Build history of the part. All positions in model axes, mm. A direction names the side the tool comes from. Round coordinates to 2 decimals unless told otherwise and drop trailing zeros. Write each loop counter-clockwise with the first axis right and the second up, starting at its lowest first coordinate (ties: lowest second). Pieces come first, ordered by that corner, then holes.
1) Which spindle directions (+Z, -Z, +X, -X, +Y, -Y) get a long thin tool onto all of the face, cutting with end or side? Do faces 1 (the flat face through (0.021, 7.127, -39.964)), 2 (the flat face through (0, 5, 2)), 3 (the flat face through (0.02, 0.58, -14.67)). Say none if no direction does.
2) Pull direction Z, two halves, no side cores. Call faces 4 (the flat face through (-1.5, 4, -14)), 5 (the cylindrical face through (-0.02, 0.07, 12.5)), 6 (the cylindrical face through (0, 0, 16)): +Z half, -Z half, draft (parallel to the pull), parting line (faces both ways), or undercut.
3) Wall check: probe 1 along Y at (x, z) = (0.1, 11); probe 2 along Z at (x, y) = (0.6, 0.5); probe 3 along Y at (x, z) = (0.35, 3). Give the ranges that are in metal, low to high.
4) Saw through at D-D (y = 3.5). Write the cut outline in (x, z), plus the area to 3 significant figures.
5) Saw through at A-A (x = -0.35). Write the cut outline in (y, z).
6) Saw through at B-B (y = 0). Write the cut outline in (x, z).
7) Flat gauge pins, fed straight in: pin 1 (3 mm diameter, centred on y = 3.5, z = -33.5, fed in from -X); pin 2 (1.5 mm diameter, centred on x = 0, y = 11, fed in from -Z); pin 3 (1.5 mm diameter, centred on x = 0.5, z = -2, fed in from +Y). Where does each tip first touch, or does it go through?
8) Saw through at C-C (z = 7.5). Write the cut outline in (x, y), plus the area to 3 significant figures.
from build123d import *

# Parameters (mm, degrees)
SKETCH1_R           = 5
SKETCH1_R_2         = 1.5
BOSS_EXTRUDE1_DEPTH = 1.5
BOSS_EXTRUDE2_DEPTH = 3
CUT_EXTRUDE1_DEPTH  = 3
CUT_EXTRUDE2_DEPTH  = 3


with BuildPart() as part:
    # Sketch1 → Boss-Extrude1 (new body, symmetric)
    with BuildSketch(Plane(origin=(0, 0, 0), x_dir=(0, 0, -1), z_dir=(1, 0, 0))):
        with BuildLine():
            ThreePointArc((-6, 0), (-7.464466094, -3.535533906), (-11, -5))
            Line((-11, -5), (11, -5))
            ThreePointArc((11, -5), (6, 0), (11, 5))
            Line((11, 5), (-11, 5))
            ThreePointArc((-11, 5), (-7.464466094, 3.535533906), (-6, 0))
        make_face()
        with Locations((-11, 0)):
            Circle(SKETCH1_R)
        with Locations((-11, 0)):
            Circle(SKETCH1_R_2, mode=Mode.SUBTRACT)
        with Locations((11, 0)):
            Circle(SKETCH1_R)
        with Locations((11, 0)):
            Circle(SKETCH1_R_2, mode=Mode.SUBTRACT)
    extrude(amount=BOSS_EXTRUDE1_DEPTH, both=True)

    # Sketch2 → Boss-Extrude2 (add)
    with BuildSketch(Plane(origin=(1.5, 0, 0), x_dir=(0, 0, -1), z_dir=(1, 0, 0))):
        with BuildLine():
            Line((34.743210425, 5.347223248), (34.979783381, 4.763328363))
            Line((34.979783381, 4.763328363), (44.247956153, 8.518454657))
            Line((44.247956153, 8.518454657), (40.196320101, 18.518454657))
            Line((40.196320101, 18.518454657), (6.830898124, 5))
            Line((6.830898124, 5), (11, 5))
            ThreePointArc((11, 5), (13.272352736, 4.453808824), (15.048249866, 2.934565218))
            Line((15.048249866, 2.934565218), (28.023691746, 8.191742029))
            Line((28.023691746, 8.191742029), (34.743210425, 5.347223248))
        make_face()
    extrude(amount=-BOSS_EXTRUDE2_DEPTH)

    # Sketch3 → Cut-Extrude1 (cut)
    with BuildSketch(Plane(origin=(1.5, 0, 0), x_dir=(0, 0, -1), z_dir=(1, 0, 0))):
        Polygon((40.196320101, 18.518454657), (35.196320101, 16.492636631), (42.222138127, 13.518454657), align=None)
    extrude(amount=-CUT_EXTRUDE1_DEPTH, mode=Mode.SUBTRACT)

    # Sketch4 → Cut-Extrude2 (cut)
    with BuildSketch(Plane(origin=(1.5, 0, 0), x_dir=(0, 0, -1), z_dir=(1, 0, 0))):
        Polygon((36.596844979, 6.098248507), (35.906600658, 5.138840993), (37.760235213, 5.889866252), align=None)
        Polygon((35.906600658, 5.138840993), (34.743210425, 5.347223248), (34.979783381, 4.763328363), align=None)
        Polygon((38.450479533, 6.849273765), (37.760235213, 5.889866252), (39.613869767, 6.64089151), align=None)
        Polygon((40.304114087, 7.600299024), (39.613869767, 6.64089151), (41.467504321, 7.391916769), align=None)
        Polygon((42.157748642, 8.351324283), (41.467504321, 7.391916769), (43.321138875, 8.142942028), align=None)
        Polygon((44.011383196, 9.102349542), (43.321138875, 8.142942028), (44.247956153, 8.518454657), align=None)
        with BuildLine():
            ThreePointArc((11, -5), (15.453808824, -2.272352736), (15.048249866, 2.934565218))
            Line((15.048249866, 2.934565218), (14.279867332, -1.844052603))
            Line((14.279867332, -1.844052603), (10.610317492, -5))
            Line((10.610317492, -5), (11, -5))
        make_face()
    extrude(amount=-CUT_EXTRUDE2_DEPTH, mode=Mode.SUBTRACT)


solid = part.part
Evaluation:
1. face 1: +X, -X, -Y
1. face 2: +Z, +X, -X, +Y
1. face 3: -Z, +X, -X, -Y
2. face 4: draft
2. face 5: undercut
2. face 6: +Z half
3. probe 1: y = -5 to -1.5, 1.5 to 5
3. probe 2: z = -14.66 to -12.41, -9.59 to 9.59, 12.41 to 15.97
3. probe 3: y = -5 to 5
4. outline: (-1.5, -16.44) - (1.5, -16.44) - (1.5, 14.57) - (-1.5, 14.57) - close
4. area: 93.0 mm2
5. outline: (-5, -10.61) - (-1.84, -14.28) - (2.93, -15.05) - (8.19, -28.02) - (5.35, -34.74) - (5.14, -35.91) - (6.1, -36.6) - (5.89, -37.76) - (6.85, -38.45) - (6.64, -39.61) - (7.6, -40.3) - (7.39, -41.47) - (8.35, -42.16) - (8.14, -43.32) - (9.1, -44.01) - (13.52, -42.22) - (16.49, -35.2) - (5, -6.83) - (5, 11) arc R5 ccw to (-5, 11) - close; hole circle Ø3 at (0, -11); hole circle Ø3 at (0, 11)
6. outline: (-1.5, -14.58) - (1.5, -14.58) - (1.5, -12.5) - (-1.5, -12.5) - close; (-1.5, -9.5) - (1.5, -9.5) - (1.5, 9.5) - (-1.5, 9.5) - close; (-1.5, 12.5) - (1.5, 12.5) - (1.5, 16) - (-1.5, 16) - close
7. pin 1: passes through
7. pin 2: stops at z = -43.55
7. pin 3: stops at y = 5
8. outline: (-1.5, -5) - (1.5, -5) - (1.5, 5) - (-1.5, 5) - close
8. area: 30.0 mm2
